Geometry check sheet. Reference: the model listing, model coordinates, mm. Round coordinates to 2 decimals unless told otherwise and drop trailing zeros. Order: outer loops, then holes, each group sorted by start corner. A loop starts at its lowest first (then second) coordinate and runs counter-clockwise, first axis right, second up. Notation, with made-up numbers: (-4, 27.25) -> (48, 27.25) arc R15 cw to (48, 52.25) -> close; hole circle Ø8 at (48.25, 80.25). An arc over 180 degrees is marked (long way). Use a Markdown table: item, result. Add a question column.
Item 1: Mould release check, pull along Y, two halves, no side actions. Record for faces 1 (the flat face through (-1.854, 77, -63)), 2 (the cylindrical face through (-3.419, -10.165, 19.192)), 3 (the cylindrical face through (-3.419, 56.532, -53.276)), 4 (the flat face through (-3.419, 27.133, -19.389)): pulls with the +Y half, pulls with the -Y half, needs draft (parallel to the pull), parting line crosses it, or undercut.
Item 2: Sectioned sample at A-A, the plane x = -4.45. State how many separate pieces and enclosed holes the cut face has, and give its area (3 significant figures).
Item 3: Material ranges on probe 1 along Z at (x, y) = (-4.8, 75); probe 2 along Z at (x, y) = (-4.1, 63.5); probe 3 along Z at (x, y) = (-3.9, 58), recorded low to high. Write a range as [from, to].
Item 4: Sectioned sample at C-C, the plane z = -29.5. Record the cut outline in (x, y), and give its area (3 significant figures).
Item 5: Gauge pin test, flat ends, axial feed: pin 1 Ø3.5 at (y, z) = (73.177, -56.25) entering from -X; pin 2 Ø1.6 at (x, y) = (-3.5, 66.5) entering from +Z. Record the tip position at first contact, or that the pin passes through.
Item 6: Sectioned sample at B-B, the plane y = 22.5. Record the cut outline in (x, z).
from build123d import *

# Parameters (mm, degrees)
SKETCH_R  = 3
PAD_DEPTH = 3.175


with BuildPart() as part:
    # Sketch (on Face26 of Binder) → Pad (new body)
    with BuildSketch(Plane.YZ.offset(-1.8542)):
        with BuildLine():
            ThreePointArc((48.931428, -55.882884), (51.137806, -61.775535), (56.923, -64.25))
            Line((56.923, -64.25), (73.608876, -64.25))
            ThreePointArc((74.457404, -64.601472), (74.068096, -64.341345), (73.608876, -64.25))
            Line((74.457404, -64.601472), (132.274816, -122.418884))
            ThreePointArc((132.626282, -123.263462), (132.534186, -122.806368), (132.274816, -122.418884))
            ThreePointArc((130.078609, -149.574244), (132.00958, -136.482484), (132.626282, -123.263462))
            ThreePointArc((130.078609, -149.574244), (136.364169, -158.981249), (145.771174, -152.695689))
            ThreePointArc((145.771174, -152.695689), (147.91132, -138.267994), (148.627, -123.7))
            ThreePointArc((148.627, -123.7), (146.152535, -117.914806), (140.259884, -115.708428))
            ThreePointArc((139.356288, -115.35822), (139.771162, -115.628595), (140.259884, -115.708428))
            Line((81.51878, -57.520712), (139.356288, -115.35822))
            ThreePointArc((81.168572, -56.617116), (81.248405, -57.105838), (81.51878, -57.520712))
            ThreePointArc((81.168572, -56.617116), (78.962194, -50.724465), (73.177, -48.25))
            Line((56.491124, -48.25), (73.177, -48.25))
            ThreePointArc((55.642596, -47.898528), (56.031904, -48.158655), (56.491124, -48.25))
            Line((55.642596, -47.898528), (-2.18522, 9.929288))
            ThreePointArc((-2.535428, 10.832884), (-2.455595, 10.344162), (-2.18522, 9.929288))
            ThreePointArc((-2.535428, 10.832884), (-10.343393, 19.197893), (-18.527, 11.2))
            ThreePointArc((-18.527, 11.2), (-18.437787, 9.384036), (-18.171009, 7.585562))
            ThreePointArc((-18.171009, 7.585562), (-14.673899, 2.43177), (-8.540693, 1.347744))
            ThreePointArc((-7.424559, 1.026492), (-7.941171, 1.331147), (-8.540693, 1.347744))
            Line((-7.424559, 1.026492), (48.58122, -54.979288))
            ThreePointArc((48.931428, -55.882884), (48.851595, -55.394162), (48.58122, -54.979288))
        make_face()
        with Locations((56.923, -56.25)):
            Circle(SKETCH_R, mode=Mode.SUBTRACT)
        with Locations((73.177, -56.25)):
            Circle(SKETCH_R, mode=Mode.SUBTRACT)
        with BuildLine():
            ThreePointArc((-13.527, 11.2), (-13.461864, 9.874122), (-13.267082, 8.561013))
            ThreePointArc((-13.267082, 8.561013), (-9.739456, 6.203928), (-7.382371, 9.731555))
            ThreePointArc((-7.527, 11.2), (-7.490755, 10.462225), (-7.382371, 9.731555))
            ThreePointArc((-7.527, 11.2), (-10.527, 14.2), (-13.527, 11.2))
        make_face(mode=Mode.SUBTRACT)
        with BuildLine():
            ThreePointArc((140.867247, -151.720238), (142.935397, -137.777908), (143.627, -123.7))
            ThreePointArc((143.627, -123.7), (140.627, -120.7), (137.627, -123.7))
            ThreePointArc((134.982536, -150.549696), (136.964288, -137.189805), (137.627, -123.7))
            ThreePointArc((134.982536, -150.549696), (137.339621, -154.077323), (140.867247, -151.720238))
        make_face(mode=Mode.SUBTRACT)
    extrude(amount=-PAD_DEPTH)


solid = part.part
Found:
| question | item | result |
|---|---|---|
| 1 | face 1 | needs draft |
| 1 | face 2 | parting line crosses it |
| 1 | face 3 | undercut |
| 1 | face 4 | pulls with the +Y half |
| 2 | separate pieces | 1 |
| 2 | enclosed holes | 4 |
| 2 | area | 2,640 mm2 |
| 3 | probe 1 | z = [-65.14, -58.63], [-53.87, -48.46] |
| 3 | probe 2 | z = [-64.25, -48.25] |
| 3 | probe 3 | z = [-64.25, -59.05], [-53.45, -48.25] |
| 4 | outline | (-5.03, 23.1) -> (-1.85, 23.1) -> (-1.85, 37.24) -> (-5.03, 37.24) -> close |
| 4 | area | 44.9 mm2 |
| 5 | pin 1 | passes through |
| 5 | pin 2 | stops at z = -48.25 |
| 6 | outline | (-5.03, -28.9) -> (-1.85, -28.9) -> (-1.85, -14.76) -> (-5.03, -14.76) -> close |
